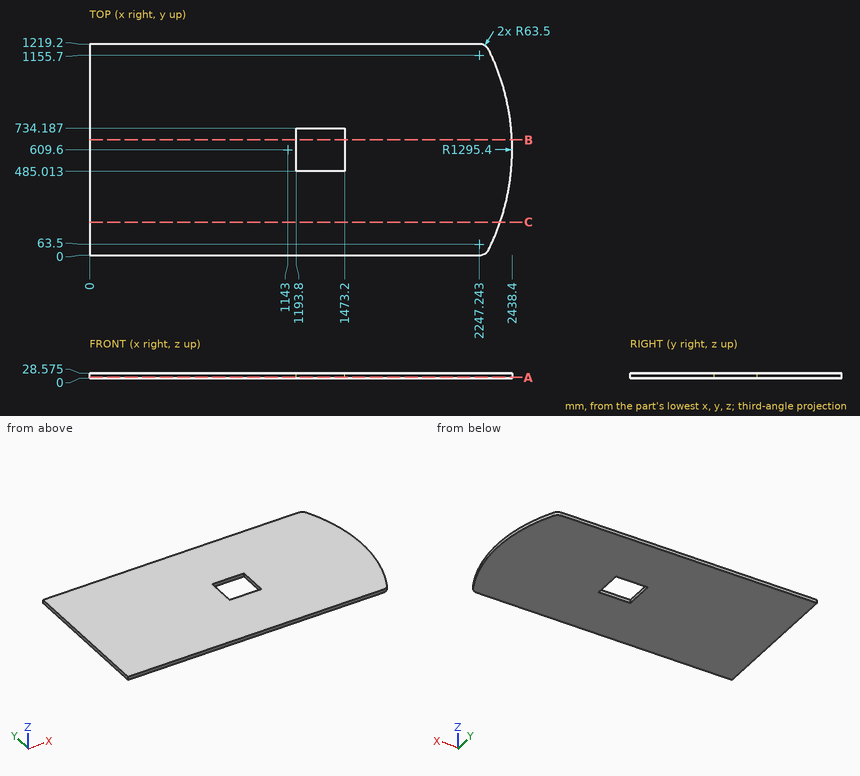
The drawing under review shows one solid part. Ordinate dimensions are in mm from its lowest x, y, z. Give positions to 0.01 mm unless a question says otherwise; leave off trailing zeros. Order: outer loops, then holes, each group sorted by start corner. A loop starts at its lowest first (then second) coordinate and runs counter-clockwise, first axis right, second up. Notation, with made-up numbers: M 72.25,3 L 124.25,3 A16 ccw 124.25,20 Z; hole C 85,70.5 d4. An arc over 180 degrees is marked long. Answer in a Markdown table with one row per item. Add a question column.
1. Add section C-C on y = 191.5. State the section outline as (x, z) points (1 decimal).
2. To check wall thickness, follow line 1 along Y through (x, z) = (1376, 13.25); line 2 along X through (y, z) = (626, 5); line 3 along X through (y, z) = (511.5, 15.5). State the ranges of each line that lie inside material, in increasing order.
3. Add section B-B on y = 666.5. State the section outline as (x, z) points (3 decimals).
4. For pin 1 Ø8 at (y, z) = (985.5, 18) entering from +X; pin 2 Ø5 at (y, z) = (283.5, 22.5) entering from +X, all flat-tipped, find the tip position at first contact; note any pin that passes through.
5. Add section A-A on z = 5.5. State the section outline as (x, y) points.
The answers:
| question | item | result |
|---|---|---|
| 1 | outline | M 0,0 L 2369.1,0 L 2369.1,28.6 L 0,28.6 Z |
| 2 | line 1 | 0 to 485.01, 734.19 to 1219.2 |
| 2 | line 2 | 0 to 1193.8, 1473.2 to 2438.3 |
| 2 | line 3 | 0 to 1193.8, 1473.2 to 2434.68 |
| 3 | outline | M 0,0 L 1193.8,0 L 1193.8,28.575 L 0,28.575 Z; M 1473.2,0 L 2437.15,0 L 2437.15,28.575 L 1473.2,28.575 Z |
| 4 | pin 1 | x = 2383.87 |
| 4 | pin 2 | x = 2397.33 |
| 5 | outline | M 0,0 L 2247.24,0 A63.5 ccw 2304.16,35.35 A1295.4 ccw 2304.16,1183.85 A63.5 ccw 2247.24,1219.2 L 0,1219.2 Z; hole M 1193.8,485.01 L 1473.2,485.01 L 1473.2,734.19 L 1193.8,734.19 Z |
